Autodesk Inventor part; units mm, degrees
ref_plane "YZ Plane" through (0, 0, 0) normal (1, 0, 0) x (0, 1, 0)
ref_plane "XZ Plane" through (0, 0, 0) normal (0, 1, 0) x (-1, 0, 0)
ref_plane "XY Plane" through (0, 0, 0) normal (0, 0, 1) x (1, 0, 0)
sketch "Sketch1" plane through (0, 0, 0) normal (0, 1, 0) x (-1, 0, 0)
  line L0 (5, 5) -> (-5, 5)
  line L1 (-5, 5) -> (-5, -5)
  line L2 (-5, -5) -> (5, -5)
  line L3 (5, -5) -> (5, 5)
  line L4 (6, 6) -> (-6, 6)
  line L5 (-6, 6) -> (-6, -6)
  line L6 (-6, -6) -> (6, -6)
  line L7 (6, -6) -> (6, 6)
  point P0 (0, 0)
  dimension "d0" = 10
  dimension "d1" = 10
  dimension "d2" = 5
  dimension "d3" = 5
  dimension "d4" = 12
  dimension "d5" = 12
  dimension "d6" = 1
  dimension "d7" = 1
extrude "Extrusion1" add sketch "Sketch1" along normal blind 2
sketch "Sketch2" plane through (6, 0, 6) normal (1, 0, 0) x (0, 0, -1)
  line L0 (0, 0) -> (0, 2)
  line L1 (12, 0) -> (12, 2)
  line L2 (0, 2) -> (12, 2)
  line L3 (12, 2) -> (12, 1)
  line L4 (12, 1) -> (0, 1)
  line L5 (0, 1) -> (0, 2)
  point P0 (6, 0)
extrude "Extrusion2" add sketch "Sketch2" against normal blind 11.5
sketch "Sketch3" plane through (0, 2, 0) normal (0, 1, 0) x (1, 0, 0)
  line L0 (-2, -2) -> (2, -2)
  line L1 (2, -2) -> (2, 2)
  line L2 (2, 2) -> (-2, 2)
  line L3 (-2, 2) -> (-2, -2)
  circle A0 centre (0, 0) radius 2.8284
  line L4 (0, -2.8284) -> (-2.8284, 0)
  line L5 (-2.8284, 0) -> (0, 2.8284)
  line L6 (2.8284, 0) -> (0, 2.8284)
  line L7 (2.8284, 0) -> (0, -2.8284)
  point P0 (0.8284, -2)
  point P1 (2, -0.8284)
  point P2 (2, 0.8284)
  point P3 (0.8284, 2)
  point P4 (-0.8284, 2)
  point P5 (-2, 0.8284)
  point P6 (-2, -0.8284)
  point P7 (-0.8284, -2)
  dimension "d13" = 4
  dimension "d14" = 4
  dimension "d15" = 2
  dimension "d16" = 2
extrude "Extrusion3" cut sketch "Sketch3" along normal blind 23.25 and the other way blind 11.625 contours L4 L3 L5 L2 L6 L1 L7 L0
sketch "Sketch4" plane through (0, 2, 0) normal (0, 1, 0) x (1, 0, 0)
  line L0 (2, -0.8284) -> (2, 0.8284)
  line L1 (2, -0.8284) -> (2.8765, -0.8284)
  line L2 (2.8765, -0.8284) -> (2.8765, 0.8284)
  line L3 (2.8765, 0.8284) -> (2, 0.8284)
  line L4 (2, 0.8284) -> (2, -0.8284)
  line L5 (2.8765, -0.8284) -> (7.5124, -0.8284)
  line L6 (7.5124, -0.8284) -> (7.5124, 0.8284)
  line L7 (7.5124, 0.8284) -> (2.8765, 0.8284)
  line L8 (2.8765, 0.8284) -> (2.8765, -0.8284)
  point P0 (0, 0)
  point P1 (2.8765, 0.8284)
  point P2 (2, 0.8284)
extrude "Extrusion4" cut sketch "Sketch4" against normal blind 1
sketch "Sketch5" plane through (0, 2, 0) normal (0, 1, 0) x (1, 0, 0)
  line L0 (-6, -6) -> (6, -6)
  line L1 (6, 0.8284) -> (6, 6)
  line L2 (-6, -6) -> (6, -6)
  line L3 (6, -6) -> (6, 6)
  line L4 (6, 6) -> (-6, 6)
  line L5 (-6, 6) -> (-6, -6)
  point P0 (0, 0)
  point P1 (6, -6)
extrude "Extrusion5" add sketch "Sketch5" along normal blind 25
sketch "Sketch6" plane through (6, 0, 6) normal (1, 0, 0) x (0, 0, -1)
  line L0 (5.1716, 1) -> (5.1716, 2)
  line L1 (5.1716, 2) -> (-3.596, 2)
  line L2 (0, 0) -> (0, 27)
  line L3 (4, 2) -> (5.1716, 2)
  line L4 (5.1716, 2) -> (16.1787, 2)
  line L5 (5.1716, 2) -> (6.8284, 2)
  line L6 (6, 2) -> (6, 6)
  line L7 (0, 2) -> (6, 4)
  line L8 (6, 4) -> (12, 2)
  line L9 (12, 0) -> (12, 27)
  line L10 (12, 2) -> (-2.4689, 2)
  line L11 (-2.4689, 2) -> (-2.4689, 28.669)
  line L12 (-2.4689, 28.669) -> (12, 28.669)
  line L13 (12, 28.669) -> (12, 2)
  point P0 (6, 0)
  dimension "d23" = 4
extrude "Extrusion6" cut sketch "Sketch6" against normal blind 23.25 contours L1 L11 L12 L13 L9 L8 L7
sketch "Sketch7" plane through (-6, 0, 6) normal (0, 0, 1) x (1, 0, 0)
  line L0 (6, 0) -> (6, 4)
  line L1 (12, 4) -> (0, 4)
  line L2 (0, 2) -> (12, 2)
  line L3 (12, 2) -> (6, 4)
  line L4 (0, 4) -> (0, 2)
  line L5 (6, 4) -> (0, 2)
  line L6 (0, 2) -> (13.6732, 2)
  line L7 (13.6732, 2) -> (13.6732, 4.9606)
  line L8 (13.6732, 4.9606) -> (0, 4.9606)
  line L9 (0, 4.9606) -> (0, 2)
extrude "Extrusion7" cut sketch "Sketch7" against normal blind 41.75 contours L5 L4 L1 | L1 L9 L8 L7 L6 L3
sketch "Sketch8" plane through (0, 2, 0) normal (0, -1, 0) x (1, 0, 0)
  line L0 (6, 6) -> (0, 0)
  line L1 (1.9974, 1.9974) -> (-2.0026, 1.9974)
  line L2 (-2.0026, 1.9974) -> (-2.0026, -2.0026)
  line L3 (-2.0026, -2.0026) -> (1.9974, -2.0026)
  line L4 (1.9974, -2.0026) -> (1.9974, 1.9974)
  dimension "d30" = 4
  dimension "d31" = 4
extrude "Extrusion8" cut sketch "Sketch8" against normal blind 105
sketch "Sketch9" plane through (6, 0, 6) normal (1, 0, 0) x (0, 0, -1)
  line L0 (0, 0) -> (0, 2)
  line L1 (12, 0) -> (12, 2)
  line L2 (0, 0) -> (12, 0)
  line L3 (12, 0) -> (12, 2)
  line L4 (12, 2) -> (0, 2)
  line L5 (0, 2) -> (0, 0)
  point P0 (6, 0)
extrude "Extrusion9" add sketch "Sketch9" along normal blind 10
sketch "Sketch10" plane through (0, 0, 0) normal (0, -1, 0) x (1, 0, 0)
  line L0 (5, -5) -> (5, 5)
  line L1 (5, 5) -> (15, 5)
  line L2 (15, 5) -> (15, -5)
  line L3 (15, -5) -> (5, -5)
  line L4 (5, -5) -> (5, 5)
  point P0 (0, 0)
  dimension "d36" = 10
extrude "Extrusion10" cut sketch "Sketch10" against normal up to surface (1 mm away)
sketch "Sketch11" plane through (6, 2, 6) normal (0, 1, 0) x (1, 0, 0)
  line L0 (10, 0) -> (10, 12)
  line L1 (0, 0) -> (-4.0026, 4.0026)
  line L2 (10, 12) -> (-4.0026, 12)
  line L3 (-4.0026, 12) -> (-4.0026, 4.0026)
  line L4 (-4.0026, 4.0026) -> (10, 4.0026)
  line L5 (10, 4.0026) -> (10, 12)
  line L6 (-12, 0) -> (10, 0)
  line L7 (-4.0026, 4.0026) -> (10, 4.0026)
  line L8 (10, 4.0026) -> (10, 0)
  line L9 (10, 0) -> (-4.0026, 0)
  line L10 (-4.0026, 0) -> (-4.0026, 4.0026)
  point P0 (-6, 6)
extrude "Extrusion11" add sketch "Sketch11" along normal blind 1.5 contours L6 L1 L4 L0 | L4 L3 L2 L0
sketch "Sketch12" plane through (16, 0, 6) normal (1, 0, 0) x (0, 0, -1)
  line L0 (0, 2) -> (12, 2)
  line L1 (4.0026, 3.3342) -> (0, 2)
  line L2 (4.0026, 2) -> (4.0026, 3.3342)
  line L3 (0, 2) -> (4.0026, 3.3342)
  line L4 (4.0026, 3.3325) -> (8.0026, 3.3325)
  line L5 (4.0026, 3.3342) -> (8.0026, 3.3325)
  line L6 (12, 0) -> (12, 2)
  line L7 (8.0026, 3.3325) -> (12, 2)
  line L8 (0, 2) -> (-1.9464, 6.2775)
  line L9 (-1.9464, 6.2775) -> (14.9869, 5.8247)
  line L10 (14.9869, 5.8247) -> (12, 2)
  point P0 (6, 0)
extrude "Extrusion12" cut sketch "Sketch12" against normal blind 26 contours L8 L9 L10 L7 L4 L1
sketch "Sketch13" plane through (-6, 0, 6) normal (0, 0, 1) x (1, 0, 0)
  line L0 (3.9974, 2) -> (3.9974, 3.3325)
  line L1 (4.0026, 3.3342) -> (0, 2)
  line L2 (3.9974, 3.3325) -> (0, 3.3325)
  line L3 (0, 3.3325) -> (0, 2)
  line L4 (0, 2) -> (3.9974, 2)
  line L5 (3.9974, 2) -> (3.9974, 3.3325)
  line L6 (22, 2) -> (0, 2)
  line L7 (22, 3.3342) -> (4.0026, 3.3342)
  line L8 (22, 2) -> (18.0026, 2)
  line L9 (18.0026, 2) -> (18.0026, 3.3342)
  line L10 (18.0026, 3.3342) -> (22, 3.3342)
  line L11 (22, 3.3342) -> (22, 2)
  line L12 (18.0026, 3.3342) -> (22, 2)
  point P0 (6, 0)
  dimension "d43" = 3.9974
  dimension "d44" = 3.9974
extrude "Extrusion13" cut sketch "Sketch13" against normal blind 17.75 contours L12 L7 L11
sketch "Sketch14" plane through (-5, 1, -5) normal (0, -1, 0) x (1, 0, 0)
  line L0 (11, 5.8284) -> (11, 4.1716)
  line L1 (11, 5.8284) -> (19.699, 5.8284)
  line L2 (19.699, 5.8284) -> (19.699, 4.1716)
  line L3 (19.699, 4.1716) -> (11, 4.1716)
  line L4 (11, 4.1716) -> (11, 5.8284)
  line L5 (19.699, 4.1716) -> (21.7329, 4.1716)
  line L6 (21.7329, 4.1716) -> (21.7329, 5.8284)
  line L7 (21.7329, 5.8284) -> (19.699, 5.8284)
  line L8 (19.699, 5.8284) -> (19.699, 4.1716)
  point P0 (5, 5)
extrude "Extrusion14" cut sketch "Sketch14" against normal up to surface (1 mm away)
sketch "Sketch15" plane through (0, 0, 0) normal (0, -1, 0) x (1, 0, 0)
  point P0 (0, 0)
sketch "Sketch16" plane through (-6, 0, -6) normal (0, 0, -1) x (-1, 0, 0)
  line L0 (-6, 0) -> (-5, 0)
  line L1 (-5, 0) -> (-5, 1.1)
  line L2 (-5, 1.1) -> (-6, 1.1)
  line L3 (-6, 1.1) -> (-6, 0)
  line L4 (-6, 0) -> (-7.1, 0)
  line L5 (-7.1, 0) -> (-7.1, 1.1)
  line L6 (-7.1, 1.1) -> (-6, 1.1)
  line L7 (-6, 1.1) -> (-6, 0)
  line L8 (-8, 1) -> (-6.8284, 1)
  line L9 (-7.1, 1) -> (-5, 1)
  line L10 (-5, 1) -> (-5, 0)
  line L11 (-5, 0) -> (-7.1, 0)
  line L12 (-7.1, 0) -> (-7.1, 1)
  point P0 (-5, 1)
  dimension "d49" = 1.1
extrude "Extrusion15" cut sketch "Sketch16" against normal blind 4.75 contours L3 L9 L1 L0 | L4 L5 L8 L9 L3
equation "\"d44\" = d43"
equation "\"BendRadius\" = Thickness"
equation "\"BendReliefWidth\" = Thickness"
equation "\"BendReliefDepth\" = 0.5 * Thickness"
equation "\"CornerReliefSize\" = 4 * Thickness"
equation "\"MinimumRemnant\" = 2 * Thickness"
equation "\"TransitionRadius\" = BendRadius"
equation "\"JacobiRadiusSize\" = BendRadius"
equation "\"GapSize\" = Thickness"
properties part number "modelGatePoklice1Prostredni"
Design review of the part built by this model. Coordinates are the model's own, in mm. A direction names the side the tool comes from. Give positions to 0.01 mm unless a question says otherwise; leave off trailing zeros. Order: outer loops, then holes, each group sorted by start corner. A loop starts at its lowest first (then second) coordinate and runs counter-clockwise, first axis right, second up.
1. Add section A-A, the plane z = -1.75. State the section outline as (x, y) points.
Solution:
outline: (-6, 0) - (-5, 0) - (-5, 1) - (-1.08, 1) - (-1.08, 2) - (-2, 2) - (-2, 3.33) - (-6, 2) - close; (1.08, 1) - (15, 1) - (15, 0) - (16, 0) - (16, 2) - (12.01, 3.33) - (2, 3.33) - (2, 2) - (1.08, 2) - close
2. To check wall thickness, follow L1, parallel to Z at x = 10.5, y = 1.25; L2, parallel to X at y = 0.35, z = 0.75; L3, parallel to Y at x = 9, z = 1.25. State the ranges of each line that lie inside material, in increasing order.
Solution:
L1: z = -6 to -0.83, 0.83 to 6
L2: x = -6 to -5, 15 to 16
L3: y = 1 to 3.33
3. For pin 1 Ø1.1 at (y, z) = (1.5, 0) entering from +X; pin 2 Ø0.5 at (x, z) = (9.5, 0.5) entering from -Y; pin 3 Ø1.1 at (x, z) = (15.5, 0) entering from +Y, all flat-tipped, find the tip position at first contact; note any pin that passes through.
Solution:
pin 1: stops at x = 16
pin 2: stops at y = 2
pin 3: stops at y = 2.35
4. Tool access review of faces 1 (the flat face through (8.1, 0.5, -5)), 2 (the flat face through (-1, 0.5, -5.5)), 3 (the flat face through (-1.42, 1.49, -1.41)), 4 (the flat face through (1.7, 2, 1.7)): name each direction out of +Z, -Z, +X, -X, +Y, -Y from which nothing blocks a thin tool from reaching the whole face with its end or side.
Solution:
face 1: -Y
face 2: -Z, -Y
face 3: +Y, -Y
face 4: +Y
5. Add section B-B, the plane y = 0.25. State the section outline as (x, z) points.
Solution:
outline: (-6, -6) - (-1, -6) - (-1, -5) - (-5, -5) - (-5, 5) - (15, 5) - (15, -5) - (1.1, -5) - (1.1, -6) - (16, -6) - (16, 6) - (-6, 6) - close
6. Add section D-D, the plane x = 8.75. State the section outline as (y, z) points, then the cut area to 3 significant figures.
Solution:
outline: (0, -6) - (2, -6) - (3.33, -2) - (3.33, 2) - (2, 6) - (0, 6) - (0, 5) - (1, 5) - (1, 0.83) - (2, 0.83) - (2, -0.83) - (1, -0.83) - (1, -5) - (0, -5) - close
area: 23.0 mm2
7. Mouldability with a two-part tool opening along Z and no side actions: class faces 5 (the flat face through (5, 1, -6)), 6 (the flat face through (9, 2, 0)), 7 (the flat face through (4.1, 0, 5.4)) as +Z half, -Z half, draft (parallel to the pull), parting line (faces both ways), or undercut.
Solution:
face 5: -Z half
face 6: undercut
face 7: draft
